```python
from build123d import *

# Parameters (mm, degrees)
BOSS_EXTRUDE2_START     = -12.7
BOSS_EXTRUDE2_DEPTH     = 12.7
F_1_4_CLEARANCE_HOLE1_D = 6.5278
CIRPATTERN3_COUNT       = 3
CHAMFER1_SIZE           = 0.635
CHAMFER1_SIZE2          = 1.744648161


with BuildPart() as part:
    # Sketch3 → Revolve1 (revolve)
    with BuildSketch(Plane(origin=(0, 0, 0), x_dir=(0, 0, -1), z_dir=(1, 0, 0)), mode=Mode.PRIVATE) as revolve1_sk:
        Polygon((0, 104.775), (23.495, 104.775), (23.495, 101.6), (20.32, 101.6), (20.32, 98.4504), (0, 98.4504), align=None)
    revolve(revolve1_sk.sketch.rotate(Axis((0, 0, 0), (0, 0, -1)), 90), axis=Axis((0, 0, 0), (0, 0, -1)))

    # Sketch8 → Boss-Extrude2 (add)
    with BuildSketch(Plane.XY.offset(BOSS_EXTRUDE2_START)):
        with BuildLine():
            ThreePointArc((-95.701964649, 65.072457101), (-104.485964967, 60.325), (-104.205383261, 50.344104028))
            ThreePointArc((-104.205383261, 50.344104028), (-101.748303649, 45.549235235), (-100.357835782, 40.343987299))
            ThreePointArc((-100.357835782, 40.343987299), (-100.041194467, 33.940544408), (-101.071009975, 27.612525556))
            ThreePointArc((-101.071009975, 27.612525556), (-90.737811682, 52.3875), (-74.448653582, 73.723799447))
            ThreePointArc((-74.448653582, 73.723799447), (-79.41397091, 69.667943629), (-85.117835782, 66.740441606))
            ThreePointArc((-85.117835782, 66.740441606), (-90.320946661, 65.341998135), (-95.701964649, 65.072457101))
        make_face()
    boss_extrude2 = extrude(amount=BOSS_EXTRUDE2_DEPTH)

    # 1/4 Clearance Hole1 (through all)
    with Locations(Plane(origin=(-78.9129789, -32.747864356, 0), x_dir=(1, 0, 0), z_dir=(0, 0, 1))):
        with Locations((-17.324094096, 88.310364356)):
            f_1_4_clearance_hole1 = Hole(F_1_4_CLEARANCE_HOLE1_D / 2)

    # CirPattern3: Boss-Extrude2, 1/4 Clearance Hole1 ×3 about axis
    cirpattern3_axis = Axis((0, 0, 0), (0, 0, 1))
    add([boss_extrude2.rotate(cirpattern3_axis, i * 360 / CIRPATTERN3_COUNT) for i in range(1, CIRPATTERN3_COUNT)])
    add([f_1_4_clearance_hole1.rotate(cirpattern3_axis, i * 360 / CIRPATTERN3_COUNT) for i in range(1, CIRPATTERN3_COUNT)], mode=Mode.SUBTRACT)

    # Chamfer1
    chamfer1_edges = [part.edges().sort_by_distance(p)[0] for p in [
        (-98.4504, 0, 0),
    ]]
    chamfer1_side = [part.faces().sort_by_distance(p)[0] for p in [
        (80.519485647, -62.098271917, 0),
    ]]
    chamfer(chamfer1_edges, length=CHAMFER1_SIZE, length2=CHAMFER1_SIZE2, reference=chamfer1_side[0])


solid = part.part
```
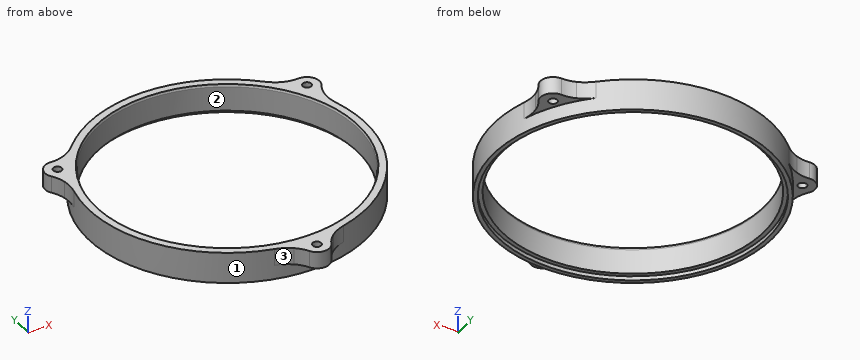
Geometry: final body of the model. Coordinates: model frame, mm. Face numbers are marked on the shaded views. Coordinates: 2 decimals unless noted, no trailing zeros. Order: outer loops, then holes, each group sorted by start corner. A loop starts at its lowest first (then second) coordinate and runs counter-clockwise, first axis right, second up. Notation, with made-up numbers: (66.25, -7) -> (70.25, -7) arc R18 ccw to (70.25, -2) -> close; hole circle Ø3 at (3.25, 89.5). An arc over 180 degrees is marked (long way). Write item = value, one per line.
(1) Cut plane B-B on z = -6.5. Count the separate pieces of the cut face and the enclosed holes in it, plus the area to 3 significant figures.
Solved:
separate_pieces = 1
enclosed_holes = 4
area = 5,020 mm²
(2) Line query: line 1 (Y direction, x = 0, z = -5.75) (3 decimals); line 2 (Y direction, x = 0, z = -21.45) (3 decimals); line 3 (Y direction, x = -2.5, z = -19.5). Output: solid intervals per line, ascending.
Solved:
line_1 = -120.65 to -114.389, -107.861 to -98.45, 98.45 to 104.775
line_2 = -104.775 to -101.6, 101.6 to 104.775
line_3 = -104.75 to -98.42, 98.42 to 104.75
(3) Cut plane A-A on y = 0. Return loops of the section in (x, z) (3 decimals).
Solved:
outline = (-104.775, -23.495) -> (-101.6, -23.495) -> (-101.6, -20.32) -> (-98.45, -20.32) -> (-98.45, -1.745) -> (-99.085, 0) -> (-104.775, 0) -> close; (98.45, -20.32) -> (101.6, -20.32) -> (101.6, -23.495) -> (104.775, -23.495) -> (104.775, 0) -> (99.085, 0) -> (98.45, -1.745) -> close
(4) Pull-direction query (X, two-part tool) for the marked faces 1, 2 and 3; classes: pulls with the +X half, pulls with the -X half, needs draft (parallel to the pull), parting line crosses it, or undercut.
Solved:
face_1 = parting line crosses it
face_2 = undercut
face_3 = pulls with the -X half
(5) Pin query (flat end, axial travel): pin 1 Ø10 at (y, z) = (-38, -16.5) entering from -X; pin 2 Ø4 at (x, z) = (27.5, -17.5) entering from -Y; pin 3 Ø2 at (x, z) = (44, -5.5) entering from +Y; pin 4 Ø6 at (x, y) = (-96.24, 55.56) entering from +Z. Return the tip coordinate at first contact, or that it passes through.
Solved:
pin_1 = -99.44
pin_2 = -101.62
pin_3 = 95.54
pin_4 = through
